Autodesk Inventor part; units mm, degrees
ref_plane "YZ Plane" through (0, 0, 0) normal (1, 0, 0) x (0, 1, 0)
ref_plane "XZ Plane" through (0, 0, 0) normal (0, 1, 0) x (-1, 0, 0)
ref_plane "XY Plane" through (0, 0, 0) normal (0, 0, 1) x (1, 0, 0)
sketch "Sketch1" plane through (0, 0, 0) normal (1, 0, 0) x (0, 1, 0)
  line L0 (0, 0) -> (50.8, 0)
  line L1 (50.8, 0) -> (50.8, -25.4)
  line L2 (50.8, -25.4) -> (0, -25.4)
  line L3 (0, -25.4) -> (0, 0)
  line L4 (49.53, -24.13) -> (49.53, -1.27)
  line L5 (49.53, -1.27) -> (1.27, -1.27)
  line L6 (1.27, -1.27) -> (1.27, -24.13)
  line L7 (1.27, -24.13) -> (49.53, -24.13)
  dimension "d0" = 50.8
  dimension "d1" = 25.4
  dimension "d2" = 1.27
extrude "Extrusion1" add sketch "Sketch1" along normal blind 609.6
sketch "Sketch2" plane through (0, 0, -25.4) normal (0, 0, -1) x (-1, 0, 0)
  circle A0 centre (-174.2245, 25.4) radius 7.3323
  circle A1 centre (-355.8783, 25.3733) radius 7.3323
  line L0 (-461.8402, 31.7005) -> (-458.3441, 31.8328)
  arc A2 (-458.0874, 31.6973) -> (-458.3441, 31.8328) centre (-461.6, 25.355) ccw
  arc A3 (-454.3512, 25.4841) -> (-454.3621, 25.7742) centre (-461.6, 25.355) ccw
  arc A4 (-457.8637, 19.1419) -> (-457.618, 19.2964) centre (-461.6, 25.355) ccw
  arc A5 (-465.3363, 31.5681) -> (-465.582, 31.4136) centre (-461.6, 25.355) ccw
  arc A6 (-468.8488, 25.2259) -> (-468.8379, 24.9358) centre (-461.6, 25.355) ccw
  arc A7 (-465.1126, 19.0127) -> (-464.8559, 18.8772) centre (-461.6, 25.355) ccw
  arc A8 (-457.8637, 19.1419) -> (-457.618, 19.2964) centre (-461.6, 25.355) ccw
  circle A9 centre (-461.8402, 25.355) radius 7.3767
  line L1 (0, 0) -> (-15.2407, 50.8)
  line L2 (0, 50.8) -> (-609.6, 50.8)
  line L3 (0, 0) -> (53.037, 0) construction
  line L4 (0, 0) -> (0, 50.8)
  line L5 (-15.2407, 50.8) -> (0, 50.8)
  dimension "d7" = 14.6647
  dimension "d9" = 106.7
extrude "Extrusion2" cut sketch "Sketch2" against normal through all
properties part number "Aluminum Channel Arm Cut"
Source: CAD feature listing. Evaluate the final solid. Frame: model axes, mm. A direction names the side the tool comes from. Coordinates: 2 decimals unless noted, no trailing zeros. Loops run counter-clockwise (first coordinate to the right, second up) from the corner with the lowest first, then second, coordinate; pieces in that order, holes last. Notation, with made-up numbers: M 60.5,53.5 L 71.5,53.5 A19 ccw 71.5,81.5 Z; hole C -29.5,7 d11. An arc over 180 degrees is marked long. Use a Markdown table: item, result. Add a question column.
Q1. Draft query along Y for faces 1 (the flat face through (301, 26, -25.4)), 2 (the cylindrical face through (349.105, 22.565, -0.644)), 3 (the flat face through (7.02, 23.4, -0.53)). Return one class per face: pulls with the +Y half, pulls with the -Y half, needs draft (parallel to the pull), parting line crosses it, or undercut.
Q2. Access query for faces 4 (the cylindrical face through (167.23, 27.6, -24.77)), 5 (the flat face through (308, 49.53, -13)). Directions: +Z, -Z, +X, -X, +Y, -Y. A direction counts if a zero-diameter tool reaches every point of the face in a straight line with its end or side. Return the directions, or none.
Q3. First-contact query: pin 1 (9 mm diameter, centred on x = 174.22, y = 25.4, fed in from +Z). Flat tip, straight axial feed; report the tip coordinate or a pass-through.
Q4. Section query C-C, the plane y = 7. Return loops of the section in (x, z), and give its area (3 significant figures).
Q5. Section query B-B, the plane x = 281. Return loops of the section in (y, z).
Q6. Section query A-A, the plane z = -6.5. Return loops of the section in (x, y).
Q7. Material intervals for L1, parallel to Z at x = 378, y = 33.5; L2, parallel to Y at x = 474, z = -7.25; L3, parallel to X at y = 44, z = -24.25, sorted ascending.
Result:
| question | item | result |
|---|---|---|
| 1 | face 1 | needs draft |
| 1 | face 2 | undercut |
| 1 | face 3 | pulls with the +Y half |
| 2 | face 4 | +Z, -Z |
| 2 | face 5 | +X, -X |
| 3 | pin 1 | passes through |
| 4 | outline | M 2.1,-25.4 L 609.6,-25.4 L 609.6,-24.13 L 2.1,-24.13 Z; M 2.1,-1.27 L 609.6,-1.27 L 609.6,0 L 2.1,0 Z |
| 4 | area | 1,540 mm2 |
| 5 | outline | M 0,-25.4 L 50.8,-25.4 L 50.8,0 L 0,0 Z; hole M 1.27,-24.13 L 49.53,-24.13 L 49.53,-1.27 L 1.27,-1.27 Z |
| 6 | outline | M 0,0 L 609.6,0 L 609.6,1.27 L 0.38,1.27 Z; M 14.86,49.53 L 609.6,49.53 L 609.6,50.8 L 15.24,50.8 Z |
| 7 | L1 | z = -25.4 to -24.13, -1.27 to 0 |
| 7 | L2 | y = 0 to 1.27, 49.53 to 50.8 |
| 7 | L3 | x = 13.2 to 609.6 |
